Autodesk Inventor part; units mm, degrees
ref_plane "YZ Plane" through (0, 0, 0) normal (1, 0, 0) x (0, 1, 0)
ref_plane "XZ Plane" through (0, 0, 0) normal (0, 1, 0) x (-1, 0, 0)
ref_plane "XY Plane" through (0, 0, 0) normal (0, 0, 1) x (1, 0, 0)
sketch "Sketch1" plane through (0, 0, 0) normal (0, 0, 1) x (1, 0, 0)
  line L0 (-75.15, 75.15) -> (75.15, 75.15)
  line L1 (75.15, 75.15) -> (75.15, -75.15)
  line L2 (75.15, -75.15) -> (-75.15, -75.15)
  line L3 (-75.15, -75.15) -> (-75.15, 75.15)
  circle A0 centre (40.4112, 40.4112) radius 3.4
  circle A1 centre (-40.4112, -40.4112) radius 3.4
  circle A2 centre (-65, 0) radius 3.35
  circle A3 centre (0, -65) radius 3.35
  circle A4 centre (0, 65) radius 3.35
  circle A5 centre (65, 0) radius 3.35
  circle A6 centre (0, 0) radius 65 construction
  circle A7 centre (0, 0) radius 37.5
  circle A8 centre (0, 0) radius 57.15 construction
  line L4 (40.4112, 40.4112) -> (-40.4112, -40.4112) construction
  point P0 (0, 75.15)
  point P1 (75.15, 0)
  dimension "d14" = 150.3
  dimension "d26" = 6.7
  dimension "d32" = 130
  dimension "d33" = 75
  dimension "d40" = 114.3
  dimension "d42" = 6.8
  dimension "d43" = 45
extrude "Extrusion1" add sketch "Sketch1" along normal blind 8
sketch "Sketch2" plane through (0, 0, 8) normal (0, 0, 1) x (1, 0, 0)
  circle A0 centre (40.4112, 40.4112) radius 3.4
  circle A1 centre (40.4112, 40.4112) radius 5.5
  circle A2 centre (-40.4112, -40.4112) radius 3.4
  circle A3 centre (-40.4112, -40.4112) radius 5.5
  point P0 (0, 0)
  dimension "d46" = 11
extrude "Extrusion2" cut sketch "Sketch2" against normal blind 6.6 contours A0 | A1 | A3
properties part number "FLI-Al-Plate" material "Aluminum 6061"
Here's how the part is built. I have some questions about the finished solid (model axes, mm). A direction names the side the tool comes from. Give positions to 0.01 mm unless a question says otherwise; leave off trailing zeros. Loops run counter-clockwise (first coordinate to the right, second up) from the corner with the lowest first, then second, coordinate; pieces in that order, holes last. Notation, with made-up numbers: (-28, 4.5) -> (-15, 4.5) arc R30 ccw to (-15, 32.5) -> close; hole circle Ø6 at (-23, 17.5). An arc over 180 degrees is marked (long way). One line per item, written item: value.
Q1. On a 3-axis mill with a long thin cutter (end or side, diameter ignored), from which of +Z, -Z, +X, -X, +Y, -Y can I reach the whole of each face in a straight line? I mean faces 1 (the face through (-43, -43, 1.4)), 2 (the face through (-0.44, -68.32, 3.94)). Say none if no direction works.
Answers follow:
face 1: +Z
face 2: +Z, -Z
Q2. We'd pull the mould along Y, two halves only. Please class faces 3 (the face through (43, 43, 1.4)), 4 (the face through (1, -75.15, 4)), 5 (the face through (-18, 34, 0)): pulls with the +Y half, pulls with the -Y half, needs draft (parallel to the pull), parting line crosses it, or undercut.
Answers follow:
face 3: undercut
face 4: pulls with the -Y half
face 5: needs draft
Q3. Suppose I cut it at A-A on x = 0. Please give me the cut outline in (y, z), then the cut area to 3 significant figures.
Answers follow:
outline: (-75.15, 0) -> (-68.35, 0) -> (-68.35, 8) -> (-75.15, 8) -> close; (-61.65, 0) -> (-37.5, 0) -> (-37.5, 8) -> (-61.65, 8) -> close; (37.5, 0) -> (61.65, 0) -> (61.65, 8) -> (37.5, 8) -> close; (68.35, 0) -> (75.15, 0) -> (75.15, 8) -> (68.35, 8) -> close
area: 495 mm^2
Q4. I'm going to push a flat-ended pin straight in: pin 1 Ø3.5 at (x, y) = (38.5, 41.5) entering from +Z. Where does the tip first touch, or does it pass through?
Answers follow:
pin 1: z = 1.4
Q5. Suppose I cut it at C-C on y = 65. Please give me the cut outline in (x, z), then the cut area to 3 significant figures.
Answers follow:
outline: (-75.15, 0) -> (-3.35, 0) -> (-3.35, 8) -> (-75.15, 8) -> close; (3.35, 0) -> (75.15, 0) -> (75.15, 8) -> (3.35, 8) -> close
area: 1,150 mm^2
Q6. If I drill on line 1 along Y through (x, z) = (-0.5, 1); line 2 along Y through (x, z) = (3.5, 3.75); line 3 along X through (y, z) = (42, 5.75), over which ranges is the centre line in solid material (lowest first)?
Answers follow:
line 1: -75.15 to -68.31, -61.69 to -37.5, 37.5 to 61.69, 68.31 to 75.15
line 2: -75.15 to -37.34, 37.34 to 75.15
line 3: -75.15 to 35.15, 45.68 to 75.15
